from build123d import *

# Parameters (mm, degrees)
F1_DEPTH = 25.4
F2_W     = 142.5245404243
F2_H     = 16.7245063931
F3_DEPTH = 5.08
F4_W     = 31.0823179224
F4_H     = 16.0704599693
F5_DEPTH = 2.286


with BuildPart() as f1:
    # F0 (on Front) → F1 (new body)
    with BuildSketch(Plane.XZ):
        with BuildLine():
            Line((17.1419177204, 27.2214487195), (-51.7388731241, 27.2214487195))
            Line((-51.7388731241, 27.2214487195), (-51.7388731241, 4.0606581606))
            Line((-51.7388731241, 4.0606581606), (-4.9744974851, -15.1898686591))
            Line((-4.9744974851, -15.1898686591), (58.3500750363, -15.1898692793))
            Line((58.3500750363, -15.1898692793), (62.2612222636, -15.1898693176))
            Line((62.2612222636, -15.1898693176), (63.4634880032, -15.1898693293))
            add(Edge.make_bspline(
                [(64.4092596529, -14.3758283739), (64.1666311948, -14.7868047997), (63.8535709364, -15.0634684427), (63.4634880032, -15.1898693293)],
                knots=[0.3722656756, 0.3722656756, 0.3722656756, 0.3722656756, 0.4188718953, 0.4188718953, 0.4188718953, 0.4188718953], degree=3))
            add(Edge.make_bspline(
                [(60.1013436317, 13.0514085218), (63.7917100626, 0.7586007856), (66.3472466315, -11.0931674362), (64.4092596529, -14.3758283739)],
                knots=[0, 0, 0, 0, 0.3722656756, 0.3722656756, 0.3722656756, 0.3722656756], degree=3))
            Line((60.1013436317, 13.0514085218), (27.1688286692, 23.1228569478))
            Line((27.1688286692, 23.1228569478), (17.1419177204, 27.2214487195))
        make_face()
        with BuildLine():
            ThreePointArc((64.4092596529, -14.3758283739), (80.818481148, 2.2534544809), (60.1013436317, 13.0514085218))
            add(Edge.make_bspline(
                [(60.1013436317, 13.0514085218), (63.7917100626, 0.7586007856), (66.3472466315, -11.0931674362), (64.4092596529, -14.3758283739)],
                knots=[0, 0, 0, 0, 0.3722656756, 0.3722656756, 0.3722656756, 0.3722656756], degree=3))
        make_face()
        with BuildLine():
            Line((63.4634880032, -15.1898693293), (62.2612222636, -15.1898693176))
            add(Edge.make_bspline(
                [(63.4634880032, -15.1898693293), (63.1173511551, -15.3020301053), (62.7105685577, -15.2958777029), (62.2612222636, -15.1898693176)],
                knots=[0.4188718953, 0.4188718953, 0.4188718953, 0.4188718953, 0.4602275369, 0.4602275369, 0.4602275369, 0.4602275369], degree=3))
        make_face()
    extrude(amount=F1_DEPTH)

    # F2 (on face) → F3 (cut)
    with BuildSketch(Plane.XY.offset(27.2214487195)):
        with Locations((12.0256319642, -13.3969103917)):
            Rectangle(F2_W, F2_H)
    extrude(amount=-F3_DEPTH, mode=Mode.SUBTRACT)

    # F4 (on face) → F5 (cut)
    with BuildSketch(Plane(origin=(8.7903255134, 0, 28.7433856833), x_dir=(0.9562806546, 0, -0.2924505251), z_dir=(0.2924505251, 0, 0.9562806546))):
        with Locations((38.115701994, -13.25293025)):
            Rectangle(F4_W, F4_H)
    extrude(amount=-F5_DEPTH, mode=Mode.SUBTRACT)


solid = f1.part
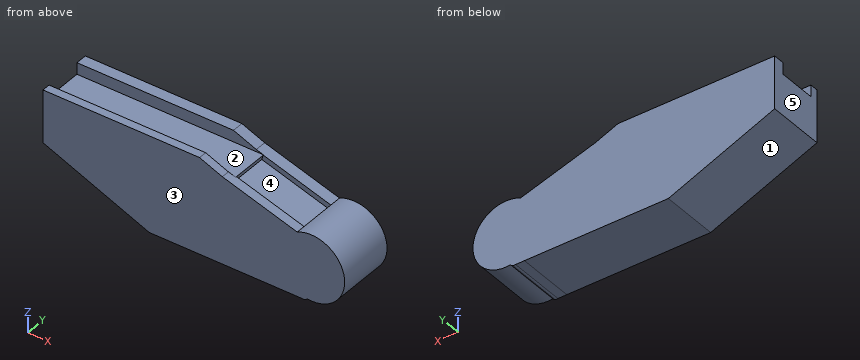
Can you work these out from the model? Positions are in its coordinate system, mm. Face numbers are marked on the shaded views. A direction names the side the tool comes from. Coordinates: 2 decimals unless noted, no trailing zeros. Write each loop counter-clockwise with the first axis right and the second up, starting at its lowest first coordinate (ties: lowest second). Pieces come first, ordered by that corner, then holes. Notation, with made-up numbers: (4, 28.5) -> (21, 28.5) arc R14 cw to (21, 54.5) -> close; hole circle Ø7 at (-15.75, 37.5). An arc over 180 degrees is marked (long way). Answer as CSV lines item,"result".
1) If I drill on line 1 (Y direction, x = 22, z = 23); line 2 (Z direction, x = 15, y = -7.25); line 3 (X direction, y = -15.75, z = 20), over which ranges is the centre line in solid material (lowest first)? Write a range as from..to.
Check result:
line 1,"-25.4..-21.76, -5.03..0"
line 2,"-15.19..22.14"
line 3,"-51.74..29.72"
2) If we section it at B-B on z = 2.5: Please give me the cut outline in (x, y), then the cut area to 3 significant figures.
Check result:
outline,"(-47.95, -25.4) -> (80.78, -25.4) -> (80.78, 0) -> (-47.95, 0) -> close"
area,"3,270 mm²"
3) Will these pins go through, and if not, where does the flat tip stop? P1, Ø6, axis at x = 23.5, y = -7, coming from the -Z side; P2, Ø6, axis at x = -16.5, y = -19, coming from the -Z side.
Check result:
P1,"z = -15.19"
P2,"z = -11.68"
4) On a 3-axis mill with a long thin cutter (end or side, diameter ignored), from which of +Z, -Z, +X, -X, +Y, -Y can I reach the whole of each face in a straight line? I mean the marked faces 1 and 2. Say none if no direction works.
Check result:
face 1,"-Z, -X, +Y, -Y"
face 2,"+Z, +X, -X"
5) If we mould it in two halves opening along X, with no side actions, what happens to the marked faces 3, 4 and 5? For each: +X half, -X half, draft (parallel to the pull), parting line (faces both ways), or undercut.
Check result:
face 3,"draft"
face 4,"undercut"
face 5,"-X half"
6) If we section it at A-A on x = 5: Please give me the cut outline in (y, z), then the cut area to 3 significant figures.
Check result:
outline,"(-25.4, -15.19) -> (0, -15.19) -> (0, 27.22) -> (-5.03, 27.22) -> (-5.03, 22.14) -> (-21.76, 22.14) -> (-21.76, 27.22) -> (-25.4, 27.22) -> close"
area,"992 mm²"
